Build history of the part. All positions in model axes, mm. Round coordinates to 2 decimals unless told otherwise and drop trailing zeros. Loops run counter-clockwise (first coordinate to the right, second up) from the corner with the lowest first, then second, coordinate; pieces in that order, holes last. Notation, with made-up numbers: M 9,78.25 L 38,78.25 A34 ccw 38,112.25 Z; hole C 45.25,27 d3. An arc over 180 degrees is marked long. One line per item, written item: value.
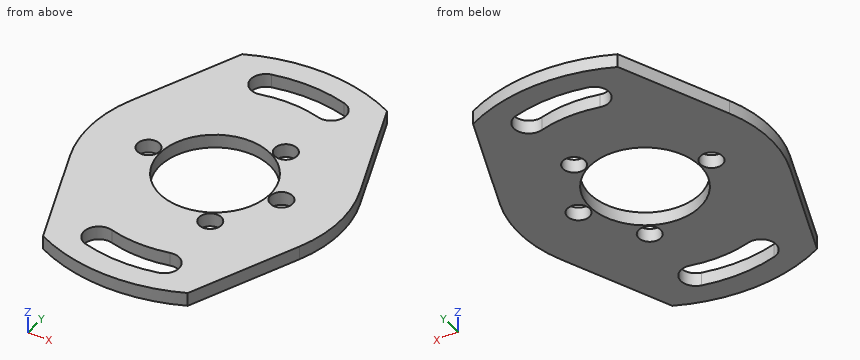
Autodesk Inventor part; units mm, degrees
ref_plane "YZ Plane" through (0, 0, 0) normal (1, 0, 0) x (0, 1, 0)
ref_plane "XZ Plane" through (0, 0, 0) normal (0, 1, 0) x (-1, 0, 0)
ref_plane "XY Plane" through (0, 0, 0) normal (0, 0, 1) x (1, 0, 0)
sketch "Эскиз1" plane through (0, 0, 0) normal (0, 0, 1) x (1, 0, 0)
  line L0 (6.9092, 5.1942) -> (2.135, 17.0596)
  arc A0 (2.135, 17.0596) -> (-14.135, 17.0596) centre (-6, 0) ccw
  line L1 (-18.9092, 5.1942) -> (-14.135, 17.0596)
  arc A1 (-18.9092, 5.1942) -> (-18.9092, -5.1942) centre (-6, 0) ccw
  line L2 (-14.135, -17.0597) -> (-18.9092, -5.1942)
  arc A2 (-14.135, -17.0597) -> (2.135, -17.0597) centre (-6, 0) ccw
  line L3 (2.135, -17.0597) -> (6.9092, -5.1942)
  arc A3 (6.9092, -5.1942) -> (6.9092, 5.1942) centre (-6, 0) ccw
  circle A4 centre (-6, 0) radius 6.1038
  arc A5 (-2.7357, 12.7023) -> (-1.9143, 15.8984) centre (-2.325, 14.3003) ccw
  arc A6 (-2.7357, 12.7023) -> (-9.2643, 12.7023) centre (-6, 0) ccw
  arc A7 (-10.0857, 15.8984) -> (-9.2643, 12.7023) centre (-9.675, 14.3003) ccw
  arc A8 (-1.9143, 15.8984) -> (-10.0857, 15.8984) centre (-6, 0) ccw
  arc A9 (-9.2643, -12.7023) -> (-10.0857, -15.8984) centre (-9.675, -14.3003) ccw
  arc A10 (-9.2643, -12.7023) -> (-2.7357, -12.7023) centre (-6, 0) ccw
  arc A11 (-1.9143, -15.8984) -> (-2.7357, -12.7023) centre (-2.325, -14.3003) ccw
  arc A12 (-10.0857, -15.8984) -> (-1.9143, -15.8984) centre (-6, 0) ccw
  circle A13 centre (-13.476, 0) radius 1.2248
  circle A14 centre (-2.2767, -6.483) radius 1.2248
  circle A15 centre (1.4761, 0) radius 1.2248
  circle A16 centre (-2.2913, 6.4913) radius 1.2248
  point P0 (0, 0)
  point P1 (-8.8708, 4.3525)
extrude "Выдавливание1" add sketch "Эскиз1" along normal blind 1.5
properties part number "Фланец"
Item 1: Slice it at D-D, the plane y = 0. Give the cut face in (x, z) (3 decimals), and give its area (3 significant figures).
Check values:
outline: M -19.915,0 L -14.701,0 L -14.701,1.5 L -19.915,1.5 Z; M -12.251,0 L -12.104,0 L -12.104,1.5 L -12.251,1.5 Z; M 0.104,0 L 0.251,0 L 0.251,1.5 L 0.104,1.5 Z; M 2.701,0 L 7.915,0 L 7.915,1.5 L 2.701,1.5 Z
area: 16.1 mm2
Item 2: Slice it at A-A, the plane x = -6. Give the cut face in (y, z) (3 decimals).
Check values:
outline: M -18.9,0 L -16.415,0 L -16.415,1.5 L -18.9,1.5 Z; M -13.115,0 L -6.104,0 L -6.104,1.5 L -13.115,1.5 Z; M 6.104,0 L 13.115,0 L 13.115,1.5 L 6.104,1.5 Z; M 16.415,0 L 18.9,0 L 18.9,1.5 L 16.415,1.5 Z
Item 3: Slice it at C-C, the plane z = 0.9. Give the cut face in (x, y) (1 decimal).
Check values:
outline: M -18.9,-5.2 L -14.1,-17.1 A18.9 ccw 2.1,-17.1 L 6.9,-5.2 A13.9 ccw 6.9,5.2 L 2.1,17.1 A18.9 ccw -14.1,17.1 L -18.9,5.2 A13.9 ccw Z; hole C -13.5,0 d2.4; hole C -6,0 d12.2; hole M -10.1,-15.9 A16.4 ccw -1.9,-15.9 A1.6 ccw -2.7,-12.7 A13.1 cw -9.3,-12.7 A1.6 ccw Z; hole M -10.1,15.9 A1.6 ccw -9.3,12.7 A13.1 cw -2.7,12.7 A1.6 ccw -1.9,15.9 A16.4 ccw Z; hole C -2.3,-6.5 d2.4; hole C -2.3,6.5 d2.4; hole C 1.5,0 d2.4
Item 4: Slice it at B-B, the plane y = -13.5. Give the cut face in (x, z), and give its area (3 significant figures).
Check values:
outline: M -15.57,0 L -11.12,0 L -11.12,1.5 L -15.57,1.5 Z; M -0.88,0 L 3.57,0 L 3.57,1.5 L -0.88,1.5 Z
area: 13.3 mm2
Item 5: Wall check: line 1 along Y through (x, z) = (-3, 0.3); line 2 along X through (y, z) = (-1, 0.55); line 3 along X through (y, z) = (5.5, 0.9). Give the ranges that are in metal, low to high.
Check values:
line 1: y = -18.66 to -16.14, -12.77 to -7.47, -5.49 to -5.32, 5.32 to 5.49, 7.49 to 12.77, 16.14 to 18.66
line 2: x = -19.88 to -14.18, -12.77 to -12.02, 0.02 to 0.77, 2.18 to 7.88
line 3: x = -18.79 to -8.65, -3.35 to -3.01, -1.57 to 6.79
